The model under review builds one solid part; all positions refer to its coordinate system, in mm. A direction names the side the tool comes from. Round coordinates to 2 decimals unless told otherwise and drop trailing zeros. Write each loop counter-clockwise with the first axis right and the second up, starting at its lowest first coordinate (ties: lowest second). Pieces come first, ordered by that corner, then holes. Notation, with made-up numbers: (-28, 74) -> (-6, 74) arc R25 ccw to (-6, 98) -> close; hole circle Ø5 at (18, 62.5). An arc over 180 degrees is marked (long way). Use CSV: the item, a comma, the result in double quotes. Start each with the question number.
1) Take a section at D-D, the plane x = -3.5. Give the boundary of the cut face in (y, z).
2) For pin 1 Ø9.5 at (x, y) = (-7.5, 3.5) entering from -Z; pin 2 Ø2.5 at (x, y) = (20, -14) entering from +Z, all flat-tipped, find the tip position at first contact; note any pin that passes through.
3) Take a section at A-A, the plane z = -1.2. State how many separate pieces and enclosed holes the cut face has, then the cut area to 3 significant figures.
4) Machinability: for faces 4 (the face through (22.797, -16.859, 0.038)), 5 (the face through (-9, 4, 1)), which of the approach directions +Z, -Z, +X, -X, +Y, -Y give a long, thin tool a straight path to every point of the face, cutting with its end or side? Answer none if there is none.
5) Take a section at B-B, the plane x = 12. Give the boundary of the cut face in (y, z), then the cut area to 3 significant figures.
6) Wall thickness on probe 1 along Y at (x, z) = (20, 0.2); probe 2 along Y at (x, z) = (-14.5, 0.65); probe 3 along Y at (x, z) = (-3.5, -1.5): over which ranges is each line inside the solid? List them lowest first. Write a range as [from, to].
7) Take a section at C-C, the plane y = 15.5. Give the boundary of the cut face in (x, z), then the cut area to 3 significant figures.
8) Mouldability with a two-part tool opening along Y and no side actions: class faces 1 (the face through (-22.797, 16.859, 0.038)), 2 (the face through (-3, 0, 1)), 3 (the face through (0, 0, 2.75)) as released by +Y, released by -Y, zero draft, split by the parting line, or undercut.
from build123d import *

# Parameters (mm, degrees)
SKETCH1_R           = 2.05
BOSS_EXTRUDE1_DEPTH = 2.75
SKETCH2_R           = 9.5
CUT_EXTRUDE1_DEPTH  = 2.5
SKETCH3_W           = 12
SKETCH3_H           = 8
CUT_EXTRUDE2_DEPTH  = 31.149626863
SKETCH4_R           = 1
CUT_EXTRUDE3_DEPTH  = 31.5
SKETCH5_W           = 6
SKETCH5_H           = 24
CUT_EXTRUDE4_DEPTH  = 31.5


with BuildPart() as part:
    # Sketch1 → Boss-Extrude1 (new, symmetric)
    with BuildSketch(Plane.XY):
        with BuildLine():
            Line((-20, -18), (20, -18))
            ThreePointArc((20, -18), (22.828427125, -16.828427125), (24, -14))
            Line((24, -14), (24, 14))
            ThreePointArc((24, 14), (22.828427125, 16.828427125), (20, 18))
            Line((20, 18), (-20, 18))
            ThreePointArc((-20, 18), (-22.828427125, 16.828427125), (-24, 14))
            Line((-24, 14), (-24, -14))
            ThreePointArc((-24, -14), (-22.828427125, -16.828427125), (-20, -18))
        make_face()
        with Locations((-20, -14)):
            Circle(SKETCH1_R, mode=Mode.SUBTRACT)
        with Locations((-20, 14)):
            Circle(SKETCH1_R, mode=Mode.SUBTRACT)
        with Locations((20, 14)):
            Circle(SKETCH1_R, mode=Mode.SUBTRACT)
        with Locations((20, -14)):
            Circle(SKETCH1_R, mode=Mode.SUBTRACT)
    extrude(amount=BOSS_EXTRUDE1_DEPTH, both=True)

    # Sketch2 → Cut-Extrude1 (cut)
    with BuildSketch(Plane.XY.offset(-2.75)):
        with Locations((-9, 0)):
            Circle(SKETCH2_R)
    extrude(amount=CUT_EXTRUDE1_DEPTH, mode=Mode.SUBTRACT)

    # Sketch3 → Cut-Extrude2 (cut, through all)
    with BuildSketch(Plane(origin=(0, 0, -0.25), x_dir=(1, 0, 0), z_dir=(0, 0, -1))):
        with Locations((-9, 0)):
            Rectangle(SKETCH3_W, SKETCH3_H)
    extrude(amount=-CUT_EXTRUDE2_DEPTH, mode=Mode.SUBTRACT)

    # Sketch4 → Cut-Extrude3 (cut, through all)
    with BuildSketch(Plane.XY.offset(2.75)):
        with Locations((-14.5, 9)):
            Circle(SKETCH4_R)
        with Locations((-3.5, 9)):
            Circle(SKETCH4_R)
        with Locations((-3.5, -9)):
            Circle(SKETCH4_R)
        with Locations((-14.5, -9)):
            Circle(SKETCH4_R)
    extrude(amount=-CUT_EXTRUDE3_DEPTH, mode=Mode.SUBTRACT)

    # Sketch5 → Cut-Extrude4 (cut, through all)
    with BuildSketch(Plane.XY.offset(2.75)):
        with Locations((12, 0)):
            Rectangle(SKETCH5_W, SKETCH5_H)
    extrude(amount=-CUT_EXTRUDE4_DEPTH, mode=Mode.SUBTRACT)


solid = part.part
Values found:
1,outline,"(-18, -2.75) -> (-10, -2.75) -> (-10, 2.75) -> (-18, 2.75) -> close; (-8, -2.75) -> (-7.75, -2.75) -> (-7.75, -0.25) -> (-4, -0.25) -> (-4, 2.75) -> (-8, 2.75) -> close; (4, -0.25) -> (7.75, -0.25) -> (7.75, -2.75) -> (8, -2.75) -> (8, 2.75) -> (4, 2.75) -> close; (10, -2.75) -> (18, -2.75) -> (18, 2.75) -> (10, 2.75) -> close"
2,pin 1,"z = -0.25"
2,pin 2,"through"
3,separate pieces,"1"
3,enclosed holes,"10"
3,area,"1,220 mm²"
4,face 4,"+Z, -Z, +X, -Y"
4,face 5,"+Z, -Z"
5,outline,"(-18, -2.75) -> (-12, -2.75) -> (-12, 2.75) -> (-18, 2.75) -> close; (12, -2.75) -> (18, -2.75) -> (18, 2.75) -> (12, 2.75) -> close"
5,area,"66.0 mm²"
6,probe 1,"[-18, -16.05], [-11.95, 11.95], [16.05, 18]"
6,probe 2,"[-18, -10], [-8, -4], [4, 8], [10, 18]"
6,probe 3,"[-18, -10], [-8, -7.75], [7.75, 8], [10, 18]"
7,outline,"(-23.71, -2.75) -> (-21.4, -2.75) -> (-21.4, 2.75) -> (-23.71, 2.75) -> close; (-18.6, -2.75) -> (18.6, -2.75) -> (18.6, 2.75) -> (-18.6, 2.75) -> close; (21.4, -2.75) -> (23.71, -2.75) -> (23.71, 2.75) -> (21.4, 2.75) -> close"
7,area,"230 mm²"
8,face 1,"released by +Y"
8,face 2,"undercut"
8,face 3,"zero draft"
